Answer from the drawing. Dimensions are ordinates in mm from the lowest x, y and z of the part. A direction names the side the tool comes from. Coordinates: 2 decimals unless noted, no trailing zeros. Write each loop counter-clockwise with the first axis right and the second up, starting at its lowest first coordinate (ties: lowest second). Pieces come first, ordered by that corner, then holes.
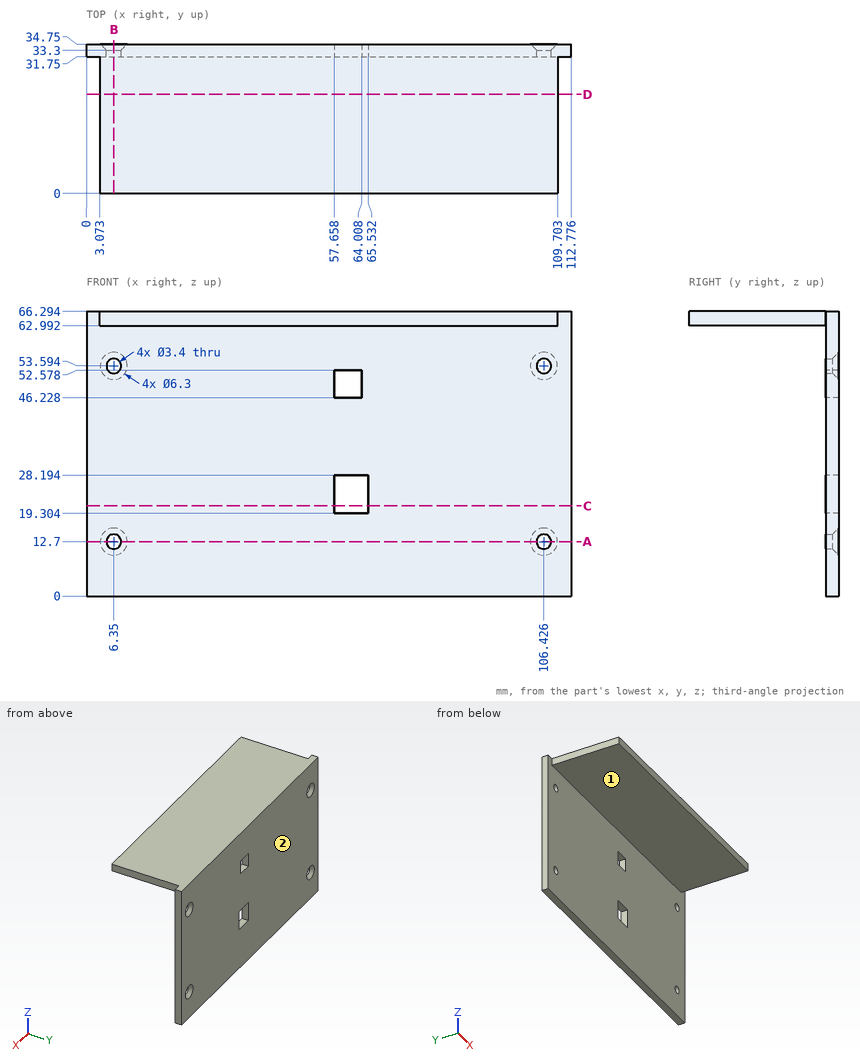
(1) Find the intervals of material crossed by probe 1 along X at (y, z) = (32.45, 12.7); probe 2 along Y at (x, z) = (5.5, 50.5); probe 3 along Z at (x, y) = (90, 22), in increasing order.
(2) Section A-A, the plane z = 12.7 is taken. Write down the section's boundary in (x, y).
(3) Section C-C, the plane z = 21 is taken. Write down the section's boundary in (x, y), plus the area to 3 significant figures.
(4) Each of these flat-tipped pins is pushed along its axis until it touches: pin 1 (0.9 mm diameter, centred on x = 63, y = 32.5, fed in from -Z); pin 2 (4 mm diameter, centred on x = 65, z = 57, fed in from -Y); pin 3 (4 mm diameter, centred on x = 106.426, z = 12.7, fed in from +Y); pin 4 (3 mm diameter, centred on x = 6.35, z = 12.7, fed in from +Y). Where does it stop, or does it pass through?
(5) Which of the six approach directions +Z, -Z, +X, -X, +Y, -Y give full straight-line access (tool end or side, diameter ignored) to the marked faces 1 and 2?
(6) Section D-D, the plane y = 23 is taken. Write down the section's boundary in (x, z), plus the area to 3 significant figures.
(7) Section B-B, the plane x = 6.35 is taken. Write down the section's boundary in (y, z).
Solution:
1. probe 1: x = 0 to 4.65, 8.05 to 104.73, 108.13 to 112.78
1. probe 2: y = 31.75 to 34.75
1. probe 3: z = 62.99 to 66.29
2. outline: (0, 31.75) - (4.65, 31.75) - (4.65, 33.3) - (3.2, 34.75) - (0, 34.75) - close; (8.05, 31.75) - (104.73, 31.75) - (104.73, 33.3) - (103.28, 34.75) - (9.5, 34.75) - (8.05, 33.3) - close; (108.13, 31.75) - (112.78, 31.75) - (112.78, 34.75) - (109.58, 34.75) - (108.13, 33.3) - close
3. outline: (0, 31.75) - (57.66, 31.75) - (57.66, 34.75) - (0, 34.75) - close; (65.53, 31.75) - (112.78, 31.75) - (112.78, 34.75) - (65.53, 34.75) - close
3. area: 315 mm2
4. pin 1: stops at z = 0
4. pin 2: stops at y = 31.75
4. pin 3: stops at y = 33.6
4. pin 4: passes through
5. face 1: -Z, +X, -X, -Y
5. face 2: +Z, -Z, +X, -X, +Y
6. outline: (3.07, 62.99) - (109.7, 62.99) - (109.7, 66.29) - (3.07, 66.29) - close
6. area: 352 mm2
7. outline: (0, 62.99) - (31.75, 62.99) - (31.75, 55.29) - (33.3, 55.29) - (34.75, 56.74) - (34.75, 66.29) - (0, 66.29) - close; (31.75, 0) - (34.75, 0) - (34.75, 9.55) - (33.3, 11) - (31.75, 11) - close; (31.75, 14.4) - (33.3, 14.4) - (34.75, 15.85) - (34.75, 50.44) - (33.3, 51.89) - (31.75, 51.89) - close
